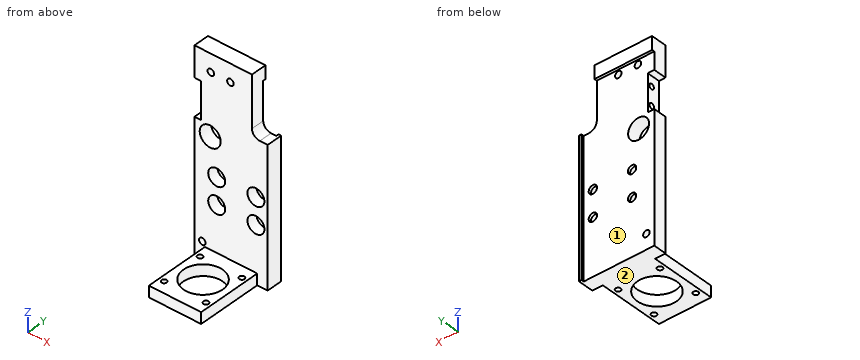
from build123d import *

# Parameters (mm, degrees)
MOUNTING_BRACKET_OUTLINE_R                     = 3.25
MOUNTING_BRACKET_OUTLINE_R_2                   = 1.25
MOUNTING_BRACKET_OUTLINE_R_3                   = 4
MOUNTING_BRACKET_DEPTH                         = 5
MOUNTING_START                                 = -25
MOUNTING_BRACKET_2_OUTLINE_W                   = 20
MOUNTING_BRACKET_2_OUTLINE_H                   = 4.25
MOUNTING_BRACKET_2_DEPTH                       = 25
MOUNTING_START_2                               = 5
MOUNTING_BRACKET_3_OUTLINE_W                   = 1
MOUNTING_BRACKET_3_OUTLINE_H                   = 52.5
MOUNTING_BRACKET_3_OUTLINE_W_2                 = 22
MOUNTING_BRACKET_3_OUTLINE_H_2                 = 5
MOUNTING_BRACKET_3_DEPTH                       = 1
MOUNTING_START_3                               = 4
MOUNTING_BRACKET_4_OUTLINE_R                   = 3.25
MOUNTING_BRACKET_4_OUTLINE_R_2                 = 1.6
MOUNTING_BRACKET_4_DEPTH                       = 1
MOUNTING_START_4                               = -4.25
MOUNTING_BRACKET_5_OUTLINE_R                   = 7.5
MOUNTING_BRACKET_5_OUTLINE_R_2                 = 0.989941464
MOUNTING_BRACKET_5_DEPTH                       = 4.25
BACK_START                                     = -25
BACK_EXTRUDE_OUTLINE_W                         = 20
BACK_EXTRUDE_OUTLINE_H                         = 4.25
BACK_EXTRUDE_DEPTH                             = 25
BACK_EXTRUDE_2_OUTLINE_R                       = 1.25
BACK_EXTRUDE_2_OUTLINE_R_2                     = 4
BACK_EXTRUDE_2_OUTLINE_R_3                     = 0.8
BACK_EXTRUDE_2_DEPTH                           = 6
BOTTOM_SKETCH_W                                = 20
BOTTOM_SKETCH_H                                = 25
BOTTOM_SKETCH_R                                = 0.989941464
BOTTOM_SKETCH_R_2                              = 7.5
BOTTOM_EXTRUDE_DEPTH                           = 4.25
CARRAIGE_MOUNT_M3S_D                           = 3.2
CARRAIGE_MOUNT_M3S_CBORE_D                     = 6.5
CARRAIGE_MOUNT_M3S_CBORE_DEPTH                 = 4
ROTATIONAL_SENSOR_TAPPED_HOLES_M2_5X0_45_D     = 2.05
ROTATIONAL_SENSOR_TAPPED_HOLES_M2_5X0_45_DEPTH = 4
ROTATIONAL_SENSOR_TAPPED_HOLES_M2_5X0_45_TIP   = 0.615882135
M3X0_5_TAPPED_HOLE1_D                          = 2.5
SKETCH5_W                                      = 27
SKETCH5_H                                      = 70
BACK_RECESS_CUT_DEPTH                          = 1


with BuildPart() as part:
    # Mounting Bracket: read off the stored shape, not the designer's step
    # Mounting Bracket outline → Mounting Bracket (new body)
    with BuildSketch(Plane(origin=(0, 0, 0), x_dir=(1, 0, 0), z_dir=(0, 1, 0))):
        with BuildLine():
            Line((14, -48.25), (14, 4.25))
            Line((14, 4.25), (-14, 4.25))
            Line((-14, 4.25), (-14, -45))
            Line((-14, -45), (-11.5, -45))
            Line((-11.5, -45), (-11.5, -59.1))
            Line((-11.5, -59.1), (-14, -59.1))
            Line((-14, -59.1), (-14, -70.75))
            Line((-14, -70.75), (8, -70.75))
            Line((8, -70.75), (8, -51.25))
            ThreePointArc((8, -51.25), (8.878679656, -49.128679656), (11, -48.25))
            Line((11, -48.25), (14, -48.25))
        make_face()
        with Locations((9.5, -17.25)):
            Circle(MOUNTING_BRACKET_OUTLINE_R, mode=Mode.SUBTRACT)
        with Locations((-7.75, -64)):
            Circle(MOUNTING_BRACKET_OUTLINE_R_2, mode=Mode.SUBTRACT)
        with Locations((-0.25, -64)):
            Circle(MOUNTING_BRACKET_OUTLINE_R_2, mode=Mode.SUBTRACT)
        with Locations((-8, -40.75)):
            Circle(MOUNTING_BRACKET_OUTLINE_R_3, mode=Mode.SUBTRACT)
        with Locations((-5.5, -27.25)):
            Circle(MOUNTING_BRACKET_OUTLINE_R, mode=Mode.SUBTRACT)
        with Locations((-5.5, -17.25)):
            Circle(MOUNTING_BRACKET_OUTLINE_R, mode=Mode.SUBTRACT)
        with Locations((-11, -1.5)):
            Circle(MOUNTING_BRACKET_OUTLINE_R_2, mode=Mode.SUBTRACT)
        with Locations((9.5, -27.25)):
            Circle(MOUNTING_BRACKET_OUTLINE_R, mode=Mode.SUBTRACT)
    extrude(amount=MOUNTING_BRACKET_DEPTH)

    # Mounting Bracket 2 outline → Mounting Bracket 2 (add)
    with BuildSketch(Plane(origin=(0, 0, 0), x_dir=(1, 0, 0), z_dir=(0, 1, 0)).offset(MOUNTING_START)):
        with Locations((0, 2.125)):
            Rectangle(MOUNTING_BRACKET_2_OUTLINE_W, MOUNTING_BRACKET_2_OUTLINE_H)
    extrude(amount=MOUNTING_BRACKET_2_DEPTH)

    # Mounting Bracket 3 outline → Mounting Bracket 3 (add)
    with BuildSketch(Plane(origin=(0, 0, 0), x_dir=(1, 0, 0), z_dir=(0, 1, 0)).offset(MOUNTING_START_2)):
        with Locations((13.5, -22)):
            Rectangle(MOUNTING_BRACKET_3_OUTLINE_W, MOUNTING_BRACKET_3_OUTLINE_H)
        with Locations((-3, -68.25)):
            Rectangle(MOUNTING_BRACKET_3_OUTLINE_W_2, MOUNTING_BRACKET_3_OUTLINE_H_2)
    extrude(amount=MOUNTING_BRACKET_3_DEPTH)

    # Mounting Bracket 4 outline → Mounting Bracket 4 (add)
    # profile 1 of 4: a face of its own
    with BuildSketch(Plane(origin=(0, 0, 0), x_dir=(1, 0, 0), z_dir=(0, 1, 0)).offset(MOUNTING_START_3)):
        with Locations((9.5, -17.25)):
            Circle(MOUNTING_BRACKET_4_OUTLINE_R)
        with Locations((9.5, -17.25)):
            Circle(MOUNTING_BRACKET_4_OUTLINE_R_2, mode=Mode.SUBTRACT)
    # profile 2 of 4: a face of its own
    with BuildSketch(Plane(origin=(0, 0, 0), x_dir=(1, 0, 0), z_dir=(0, 1, 0)).offset(MOUNTING_START_3)):
        with Locations((-5.5, -17.25)):
            Circle(MOUNTING_BRACKET_4_OUTLINE_R)
        with Locations((-5.5, -17.25)):
            Circle(MOUNTING_BRACKET_4_OUTLINE_R_2, mode=Mode.SUBTRACT)
    # profile 3 of 4: a face of its own
    with BuildSketch(Plane(origin=(0, 0, 0), x_dir=(1, 0, 0), z_dir=(0, 1, 0)).offset(MOUNTING_START_3)):
        with Locations((-5.5, -27.25)):
            Circle(MOUNTING_BRACKET_4_OUTLINE_R)
        with Locations((-5.5, -27.25)):
            Circle(MOUNTING_BRACKET_4_OUTLINE_R_2, mode=Mode.SUBTRACT)
    # profile 4 of 4: a face of its own
    with BuildSketch(Plane(origin=(0, 0, 0), x_dir=(1, 0, 0), z_dir=(0, 1, 0)).offset(MOUNTING_START_3)):
        with Locations((9.5, -27.25)):
            Circle(MOUNTING_BRACKET_4_OUTLINE_R)
        with Locations((9.5, -27.25)):
            Circle(MOUNTING_BRACKET_4_OUTLINE_R_2, mode=Mode.SUBTRACT)
    extrude(amount=MOUNTING_BRACKET_4_DEPTH)

    # Mounting Bracket 5 outline → Mounting Bracket 5 (cut)
    with BuildSketch(Plane.XY.offset(MOUNTING_START_4)):
        with Locations((0, -12.5)):
            Circle(MOUNTING_BRACKET_5_OUTLINE_R)
        with Locations((-8, -4.5)):
            Circle(MOUNTING_BRACKET_5_OUTLINE_R_2)
        with Locations((8, -4.5)):
            Circle(MOUNTING_BRACKET_5_OUTLINE_R_2)
        with Locations((8, -20.5)):
            Circle(MOUNTING_BRACKET_5_OUTLINE_R_2)
        with Locations((-8, -20.5)):
            Circle(MOUNTING_BRACKET_5_OUTLINE_R_2)
    extrude(amount=MOUNTING_BRACKET_5_DEPTH, mode=Mode.SUBTRACT)

    # Mounting Bracket 6 outline → Mounting Bracket 6 (revolve, cut)
    with BuildSketch(Plane(origin=(0, 3.25, 48.25), x_dir=(0, 1, 0), z_dir=(0, 0, -1))):
        Polygon((1.025, -7.5), (0, -6.884117865), (0, -11.5), (1.025, -11.5), align=None)
    revolve(axis=Axis((0, 3.25, 48.25), (1, 0, 0)), mode=Mode.SUBTRACT)

    # Mounting Bracket 7 outline → Mounting Bracket 7 (revolve, cut)
    with BuildSketch(Plane(origin=(0, 3.25, 55.25), x_dir=(0, 1, 0), z_dir=(0, 0, -1))):
        Polygon((1.025, -7.5), (0, -6.884117865), (0, -11.5), (1.025, -11.5), align=None)
    revolve(axis=Axis((0, 3.25, 55.25), (1, 0, 0)), mode=Mode.SUBTRACT)

    # Back Extrude: read off the stored shape, not the designer's step
    # Back Extrude outline → Back Extrude (cut)
    with BuildSketch(Plane(origin=(0, 0, 0), x_dir=(1, 0, 0), z_dir=(0, 1, 0)).offset(BACK_START)):
        with Locations((0, 2.125)):
            Rectangle(BACK_EXTRUDE_OUTLINE_W, BACK_EXTRUDE_OUTLINE_H)
    extrude(amount=BACK_EXTRUDE_DEPTH, mode=Mode.SUBTRACT)

    # Back Extrude 2 outline → Back Extrude 2 (add)
    with BuildSketch(Plane(origin=(0, 0, 0), x_dir=(1, 0, 0), z_dir=(0, 1, 0))):
        with BuildLine():
            Line((11, -48.25), (13, -48.25))
            Line((13, -48.25), (13, 4.25))
            Line((13, 4.25), (-14, 4.25))
            Line((-14, 4.25), (-14, -45))
            Line((-14, -45), (-11.5, -45))
            Line((-11.5, -45), (-11.5, -59.1))
            Line((-11.5, -59.1), (-14, -59.1))
            Line((-14, -59.1), (-14, -65.75))
            Line((-14, -65.75), (8, -65.75))
            Line((8, -65.75), (8, -51.25))
            ThreePointArc((8, -51.25), (8.878679656, -49.128679656), (11, -48.25))
        make_face()
        with Locations((-7.75, -64)):
            Circle(BACK_EXTRUDE_2_OUTLINE_R, mode=Mode.SUBTRACT)
        with Locations((-8, -40.75)):
            Circle(BACK_EXTRUDE_2_OUTLINE_R_2, mode=Mode.SUBTRACT)
        with Locations((-0.25, -64)):
            Circle(BACK_EXTRUDE_2_OUTLINE_R, mode=Mode.SUBTRACT)
        with Locations((-5.5, -27.25)):
            Circle(BACK_EXTRUDE_2_OUTLINE_R_3, mode=Mode.SUBTRACT)
        with Locations((-5.5, -17.25)):
            Circle(BACK_EXTRUDE_2_OUTLINE_R_3, mode=Mode.SUBTRACT)
        with Locations((9.5, -27.25)):
            Circle(BACK_EXTRUDE_2_OUTLINE_R_3, mode=Mode.SUBTRACT)
        with Locations((9.5, -17.25)):
            Circle(BACK_EXTRUDE_2_OUTLINE_R_3, mode=Mode.SUBTRACT)
    extrude(amount=BACK_EXTRUDE_2_DEPTH)

    # Bottom Sketch → Bottom Extrude (add)
    with BuildSketch(Plane.XY):
        with Locations((0, -12.5)):
            Rectangle(BOTTOM_SKETCH_W, BOTTOM_SKETCH_H)
        with Locations((-8, -20.5)):
            Circle(BOTTOM_SKETCH_R, mode=Mode.SUBTRACT)
        with Locations((8, -20.5)):
            Circle(BOTTOM_SKETCH_R, mode=Mode.SUBTRACT)
        with Locations((-8, -4.5)):
            Circle(BOTTOM_SKETCH_R, mode=Mode.SUBTRACT)
        with Locations((0, -12.5)):
            Circle(BOTTOM_SKETCH_R_2, mode=Mode.SUBTRACT)
        with Locations((8, -4.5)):
            Circle(BOTTOM_SKETCH_R, mode=Mode.SUBTRACT)
    extrude(amount=-BOTTOM_EXTRUDE_DEPTH)

    # Carraige Mount M3s (through all)
    with Locations(Plane(origin=(9.5, 0, 27.25), x_dir=(0, 0, -1), z_dir=(0, -1, 0))):
        with Locations((0, 0), (0, -15), (10, -15), (10, 0)):
            CounterBoreHole(CARRAIGE_MOUNT_M3S_D / 2, CARRAIGE_MOUNT_M3S_CBORE_D / 2, CARRAIGE_MOUNT_M3S_CBORE_DEPTH)

    # Rotational Sensor Tapped Holes M2.5x0.45
    with Locations(Plane.ZY.offset(11.5)):
        with Locations((55.25, 3.25), (48.25, 3.25)):
            Hole(ROTATIONAL_SENSOR_TAPPED_HOLES_M2_5X0_45_D / 2, depth=ROTATIONAL_SENSOR_TAPPED_HOLES_M2_5X0_45_DEPTH)
            with Locations((0, 0, -(ROTATIONAL_SENSOR_TAPPED_HOLES_M2_5X0_45_DEPTH + ROTATIONAL_SENSOR_TAPPED_HOLES_M2_5X0_45_TIP / 2))):  # 118° drill point
                Cone(0, ROTATIONAL_SENSOR_TAPPED_HOLES_M2_5X0_45_D / 2, ROTATIONAL_SENSOR_TAPPED_HOLES_M2_5X0_45_TIP, mode=Mode.SUBTRACT)

    # M3x0.5 Tapped Hole1 (through all)
    with Locations(Plane(origin=(0, 6, 0), x_dir=(1, 0, 0), z_dir=(0, 1, 0))):
        with Locations((-11, -1.5)):
            Hole(M3X0_5_TAPPED_HOLE1_D / 2)

    # Sketch5 → Back Recess Cut (cut)
    with BuildSketch(Plane(origin=(0, 6, 0), x_dir=(1, 0, 0), z_dir=(0, 1, 0))):
        with Locations((-0.5, -30.75)):
            Rectangle(SKETCH5_W, SKETCH5_H)
    extrude(amount=-BACK_RECESS_CUT_DEPTH, mode=Mode.SUBTRACT)


solid = part.part
Geometry check sheet. Reference: the model listing, model coordinates, mm. Face numbers are marked on the shaded views. A direction names the side the tool comes from. Give positions to 0.01 mm unless a question says otherwise; leave off trailing zeros. Write each loop counter-clockwise with the first axis right and the second up, starting at its lowest first coordinate (ties: lowest second). Pieces come first, ordered by that corner, then holes. Notation, with made-up numbers: M 55.25,74.5 L 71.25,74.5 A16 cw 71.25,97.5 Z; hole C 30,76.25 d11. An arc over 180 degrees is marked long. One line per question, with ' | ' between items.
1. Set-up check for the marked faces 1 and 2: record each of +Z, -Z, +X, -X, +Y, -Y from which the full face is reachable in a straight line by a thin tool's end or side.
Ans:
face 1: -Z, -X, +Y | face 2: -Z, +X, -X, +Y, -Y
2. Cross-section at D-D (x = 5.5). Enter the section's corners in (y, z), plus the area to 3 significant figures.
Ans:
outline: M -25,-4.25 L -17.6,-4.25 L -17.6,0 L -25,0 Z; M -7.4,-4.25 L 5,-4.25 L 5,65.75 L 6,65.75 L 6,70.75 L 0,70.75 L 0,0 L -7.4,0 Z | area: 443 mm2
3. Scan lines: line 1 along X through (y, z) = (4.75, 17.25); line 2 along Y through (x, z) = (-8, -2.75); line 3 along Z through (x, y) = (-10, 1). Record each from-to range of solid material in increasing order. Write a range as from..to.
Ans:
line 1: -14..-7.1, -3.9..7.9, 11.1..14 | line 2: -25..-21.49, -19.51..-5.49, -3.51..5 | line 3: -4.25..0.75, 2.25..37.29, 44.21..70.75
4. Cross-section at B-B (y = -18). Enter the section's corners in (x, z), plus the area to 3 significant figures.
Ans:
outline: M -10,-4.25 L -5.1,-4.25 L -5.1,0 L -10,0 Z; M 5.1,-4.25 L 10,-4.25 L 10,0 L 5.1,0 Z | area: 41.7 mm2
5. Gauge pin test, flat ends, axial feed: pin 1 (2.5 mm diameter, centred on x = 12, y = 3.5, fed in from +Z); pin 2 (8.5 mm diameter, centred on x = -0.5, z = 51.5, fed in from -Y); pin 3 (4 mm diameter, centred on x = -5.5, z = 17.25, fed in from -Y). Record the tip position at first contact, or that the pin passes through.
Ans:
pin 1: z = 48.26 | pin 2: y = 0 | pin 3: y = 4
6. Cross-section at C-C (z = 64). Enter the section's corners in (x, y).
Ans:
outline: M -14,0 L -9,0 L -9,5 L -14,5 Z; M -6.5,0 L -1.5,0 L -1.5,5 L -6.5,5 Z; M 1,0 L 8,0 L 8,5 L 1,5 Z
7. Cross-section at A-A (z = 1.5). Enter the section's corners in (x, y), plus the area to 4 significant figures.
Ans:
outline: M -14,0 L -12.25,0 L -12.25,5 L -14,5 Z; M -9.75,0 L 14,0 L 14,6 L 13,6 L 13,5 L -9.75,5 Z | area: 128.5 mm2
